Could you check a few things on this model? Use its own coordinates, in mm. Face numbers are marked on the shaded views. Give positions to 0.01 mm unless a question says otherwise; leave off trailing zeros. Order: outer loops, then holes, each group sorted by start corner. A loop starts at its lowest first (then second) coordinate and runs counter-clockwise, first axis right, second up. Notation, with made-up numbers: M 77.5,50 L 119.5,50 A26 cw 119.5,83 Z; hole C 52.5,0.5 d10. An arc over 180 degrees is marked long. Answer in a Markdown table with one row per item. Add a question column.
```python
from build123d import *

# Parameters (mm, degrees)
F0_W     = 72
F0_H     = 65
F0_R     = 15
F1_DEPTH = 10
F5_DEPTH = 5


with BuildPart() as f1:
    # F0 (on Top) → F1 (new body)
    with BuildSketch(Plane.XY):
        Rectangle(F0_W, F0_H)
        Circle(F0_R, mode=Mode.SUBTRACT)
    extrude(amount=F1_DEPTH)

    # F2 (on Right) → F3 (revolve, cut)
    with BuildSketch(Plane.YZ):
        Polygon((-20.1, 0), (0, 0), (0, 5), (-21.6, 5), (-20.1, 1), align=None)
    revolve(axis=Axis((0, 0, 2.5), (0, 0, -1)), mode=Mode.SUBTRACT)

    # F4 (on face) → F5 (cut)
    with BuildSketch(Plane(origin=(0, 0, 0), x_dir=(1, 0, 0), z_dir=(0, 0, -1))):
        with BuildLine():
            ThreePointArc((0, 21.6), (-15.273506, 15.273506), (-21.6, 0))
            Line((-21.6, 0), (-20.1, 0))
            ThreePointArc((-20.1, 0), (-14.212846, 14.212846), (0, 20.1))
            Line((0, 20.1), (0, 21.6))
        make_face()
        with BuildLine():
            Line((0, -20.1), (0, -21.6))
            ThreePointArc((0, -21.6), (15.273506, -15.273506), (21.6, 0))
            Line((21.6, 0), (20.1, 0))
            ThreePointArc((20.1, 0), (14.212846, -14.212846), (0, -20.1))
        make_face()
    extrude(amount=-F5_DEPTH, mode=Mode.SUBTRACT)


solid = f1.part
```
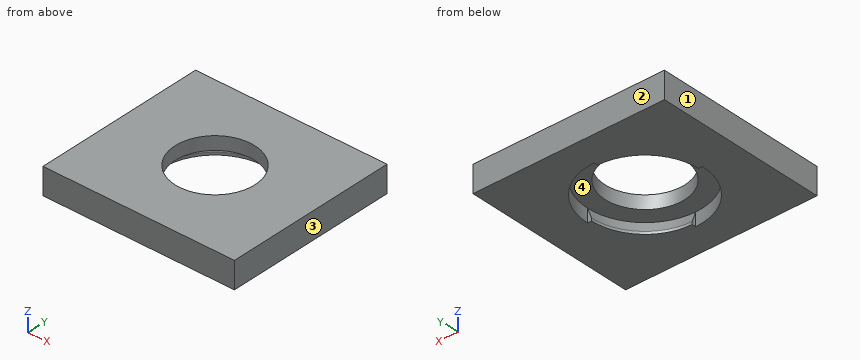
1. Suppose I cut it at A-A on z = 6.75. List the corners of the cut face in (x, y) for me, plus the area to 3 significant figures.
2. If I drill on line 1 along Y through (x, z) = (0, 8.15); line 2 along X through (y, z) = (0, 7.3); line 3 along Z through (x, y) = (17.5, -7), over which ranges is the centre line in solid material (lowest first)? Write a range as [from, to].
3. Thinking about a two-plate mould opening in X: for the marked faces 1, 2, 3 and 4, which applies, pulls with the +X half, pulls with the -X half, needs draft (parallel to the pull), parting line crosses it, or undercut?
4. Will this pin go through, and if not, where does the flat tip stop? P1, Ø21.5, axis at x = -3, y = -9, coming from the -Z side.
5. Suppose I cut it at B-B on z = 2. List the corners of the cut face in (x, y) for me (3 decimals), plus the area to 3 significant figures.
Findings below:
| question | item | result |
|---|---|---|
| 1 | outline | M -36,-32.5 L 36,-32.5 L 36,32.5 L -36,32.5 Z; hole C 0,0 d30 |
| 1 | area | 3,970 mm2 |
| 2 | line 1 | [-32.5, -15], [15, 32.5] |
| 2 | line 2 | [-36, -15], [15, 36] |
| 2 | line 3 | [5, 10] |
| 3 | face 1 | pulls with the -X half |
| 3 | face 2 | needs draft |
| 3 | face 3 | pulls with the +X half |
| 3 | face 4 | undercut |
| 4 | P1 | z = 5 |
| 5 | outline | M -36,-32.5 L 36,-32.5 L 36,32.5 L -36,32.5 Z; hole M -21.6,0 A21.6 ccw 0,-21.6 L 0,-20.475 A20.475 ccw 20.475,0 L 21.6,0 A21.6 ccw 0,21.6 L 0,20.475 A20.475 ccw -20.475,0 Z |
| 5 | area | 3,290 mm2 |
